Build history of the part. All positions in model axes, mm. Give positions to 0.01 mm unless a question says otherwise; leave off trailing zeros. Write each loop counter-clockwise with the first axis right and the second up, starting at its lowest first coordinate (ties: lowest second). Pieces come first, ordered by that corner, then holes. Notation, with made-up numbers: (19, 44.25) -> (28, 44.25) arc R28 ccw to (28, 62.25) -> close; hole circle Ø10 at (84, 32.25). An arc over 180 degrees is marked (long way). Put each result on its own line as item: value. Start each with the question number.
Item 1: Flat gauge pins, fed straight in: pin 1 Ø1 at (x, z) = (-178.5, 0) entering from -Y; pin 2 Ø4.5 at (x, y) = (102.5, 17.5) entering from -Z; pin 3 Ø2 at (y, z) = (-42, -0.5) entering from -X; pin 4 Ø2 at (y, z) = (-43, -1) entering from +X. Where does each tip first touch, or does it go through?
Item 2: Slice it at B-B, the plane x = 67.5. List the corners of the cut face in (y, z), plus the area to 3 significant figures.
Item 3: Drill centre lines: line 1 along X through (y, z) = (17, -1); line 2 along Y through (x, z) = (102.5, -0.7); line 3 along Y through (x, z) = (302.5, 0.4). Where is each one in solid material? Low to high.
Item 4: Slice it at A-A, the plane z = 0.55. List the corners of the cut face in (x, y), plus the area to 3 significant figures.
```python
from build123d import *

# Parameters (mm, degrees)
SKETCH_1_W          = 670
SKETCH_1_H          = 95
EXTRUDE_1_DEPTH     = 2
SKETCH_2_W          = 125
SKETCH_2_H          = 12.454397838
CUT_EXTRUDE_1_DEPTH = 339.374422792
SKETCH_5_R          = 2.5
CUT_EXTRUDE_4_DEPTH = 339.374422792


with BuildPart() as part:
    # Эскиз1 → Бобышка-Вытянуть1 (new, symmetric)
    with BuildSketch(Plane.XY):
        Rectangle(SKETCH_1_W, SKETCH_1_H)
    extrude(amount=EXTRUDE_1_DEPTH, both=True)

    # Эскиз2 → Вырез-Вытянуть1 (cut, through all)
    with BuildSketch(Plane.XY.offset(2)):
        with Locations((-372.5, -41.272801081)):
            Rectangle(SKETCH_2_W, SKETCH_2_H)
        with Locations((-223.5, -41.272801081)):
            Rectangle(SKETCH_2_W, SKETCH_2_H)
        with Locations((-74.5, -41.272801081)):
            Rectangle(SKETCH_2_W, SKETCH_2_H)
        with Locations((74.5, -41.272801081)):
            Rectangle(SKETCH_2_W, SKETCH_2_H)
        with Locations((223.5, -41.272801081)):
            Rectangle(SKETCH_2_W, SKETCH_2_H)
        with Locations((372.5, -41.272801081)):
            Rectangle(SKETCH_2_W, SKETCH_2_H)
    extrude(amount=-CUT_EXTRUDE_1_DEPTH, mode=Mode.SUBTRACT)

    # Эскиз5 → Вырез-Вытянуть4 (cut, through all)
    with BuildSketch(Plane.XY.offset(2)):
        with Locations((-102.5, 17.5)):
            Circle(SKETCH_5_R)
        with Locations((102.5, 17.5)):
            Circle(SKETCH_5_R)
        with Locations((-302.5, 17.5)):
            Circle(SKETCH_5_R)
        with Locations((302.5, 17.5)):
            Circle(SKETCH_5_R)
    extrude(amount=-CUT_EXTRUDE_4_DEPTH, mode=Mode.SUBTRACT)


solid = part.part
```
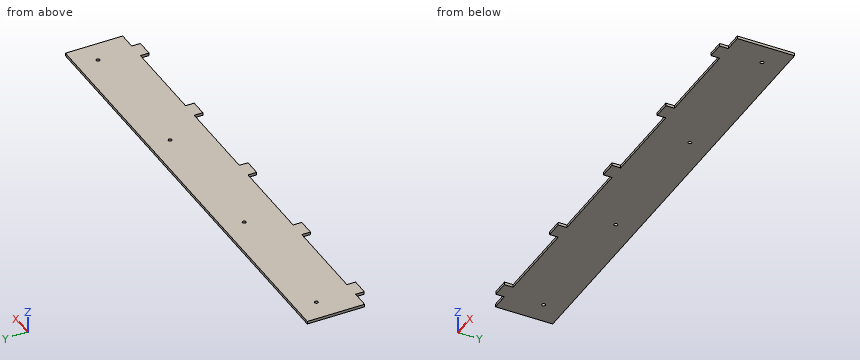
Values follow:
1. pin 1: y = -35.05
1. pin 2: through
1. pin 3: x = -310
1. pin 4: x = 310
2. outline: (-35.05, -2) -> (47.5, -2) -> (47.5, 2) -> (-35.05, 2) -> close
2. area: 330 mm2
3. line 1: -335 to -304.95, -300.05 to -104.95, -100.05 to 100.05, 104.95 to 300.05, 304.95 to 335
3. line 2: -35.05 to 15, 20 to 47.5
3. line 3: -47.5 to 15, 20 to 47.5
4. outline: (-335, -35.05) -> (-310, -35.05) -> (-310, -47.5) -> (-286, -47.5) -> (-286, -35.05) -> (-161, -35.05) -> (-161, -47.5) -> (-137, -47.5) -> (-137, -35.05) -> (-12, -35.05) -> (-12, -47.5) -> (12, -47.5) -> (12, -35.05) -> (137, -35.05) -> (137, -47.5) -> (161, -47.5) -> (161, -35.05) -> (286, -35.05) -> (286, -47.5) -> (310, -47.5) -> (310, -35.05) -> (335, -35.05) -> (335, 47.5) -> (-335, 47.5) -> close; hole circle Ø5 at (-302.5, 17.5); hole circle Ø5 at (-102.5, 17.5); hole circle Ø5 at (102.5, 17.5); hole circle Ø5 at (302.5, 17.5)
4. area: 56,700 mm2
